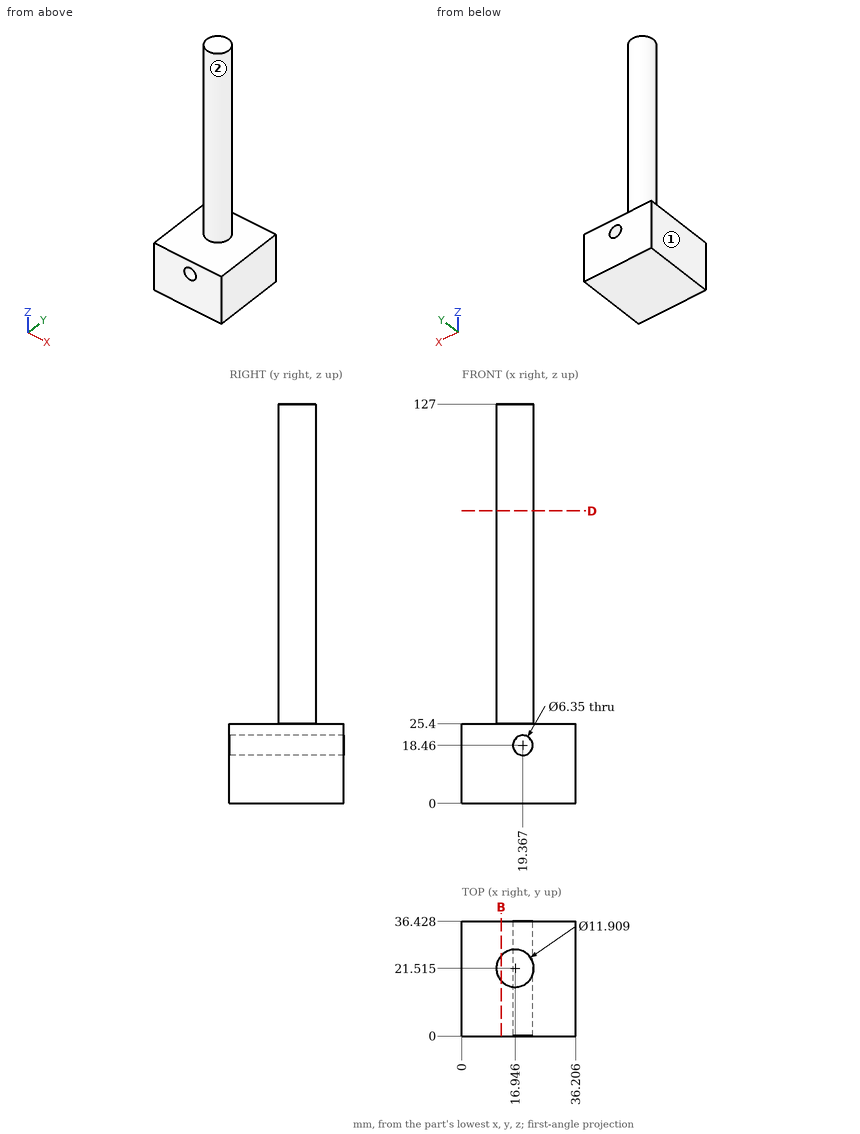
Geometry check sheet. Reference: drawing and pictorial views, mm from the part's lowest x, y, z. A direction names the side the tool comes from. Round coordinates to 2 decimals unless told otherwise and drop trailing zeros. Loops run counter-clockwise (first coordinate to the right, second up) from the corner with the lowest first, then second, coordinate; pieces in that order, holes last. Notation, with made-up numbers: (-22, -22) -> (6, -22) arc R36 cw to (6, 12) -> close; hole circle Ø9 at (-28.75, 58.25). An arc over 180 degrees is marked (long way). Answer as a JSON object with one key per item and string values. Group by question number.
Item 1: Depth check by flat-ended pin: pin 1 Ø2 at (x, z) = (17, 67.5) entering from -Y; pin 2 Ø4 at (y, z) = (19, 43) entering from -X; pin 3 Ø4 at (x, y) = (31.5, 32.5) entering from +Z. Enter the tip coordinate at first touch or a pass-through.
Item 2: Thickness scan on line 1 along Z through (x, y) = (19, 4.5) (1 decimal); line 2 along Z through (x, y) = (14.5, 15.5); line 3 along Y through (x, z) = (13.5, 109). Record the ranges inside material, lowest first.
Item 3: Set-up check for the marked faces 1 and 2: record each of +Z, -Z, +X, -X, +Y, -Y from which the full face is reachable in a straight line by a thin tool's end or side.
Item 4: Cross-section at B-B, the plane x = 12.5. Record the cut outline in (y, z) (1 decimal), plus the area to 3 significant figures.
Item 5: Cross-section at D-D, the plane z = 93. Record the cut outline in (x, y) (1 decimal).
Determined:
{
 "1": {"pin 1": "stops at y = 15.56", "pin 2": "stops at x = 11.01", "pin 3": "stops at z = 25.4"},
 "2": {"line 1": "z = 0 to 15.3, 21.6 to 25.4", "line 2": "z = 0 to 25.4", "line 3": "y = 16.66 to 26.37"},
 "3": {"face 1": "+Z, -Z, -X, +Y, -Y", "face 2": "+Z"},
 "4": {"outline": "(0, 0) -> (36.4, 0) -> (36.4, 25.4) -> (25.5, 25.4) -> (25.5, 127) -> (17.6, 127) -> (17.6, 25.4) -> (0, 25.4) -> close", "area": "1,730 mm²"},
 "5": {"outline": "circle Ø11.9 at (16.9, 21.5)"}
}
